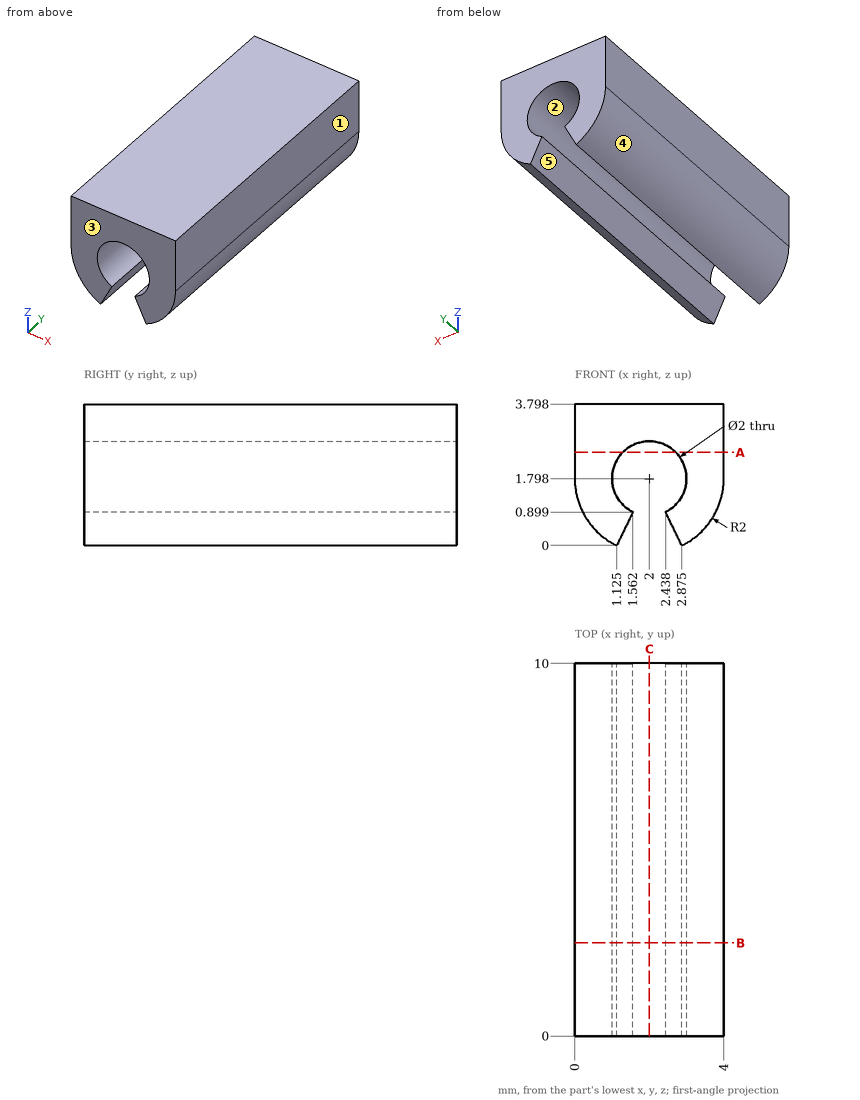
Print and shaded views of the part. All mm, measured from the part's lowest x, y and z. A direction names the side the tool comes from. Coordinates: 2 decimals unless noted, no trailing zeros. Loops run counter-clockwise (first coordinate to the right, second up) from the corner with the lowest first, then second, coordinate; pieces in that order, holes last. Notation, with made-up numbers: (22.25, 84.5) -> (57.25, 84.5) arc R27 ccw to (57.25, 107.5) -> close; hole circle Ø1 at (72, -8.75). An arc over 180 degrees is marked (long way). Use a Markdown table: item, result. Add a question column.
Item 1: Band-saw the part on B-B on y = 2.5. Write the cut outline in (x, z) (1 decimal).
Item 2: Band-saw the part on C-C on x = 2. Write the cut outline in (y, z).
Item 3: Probe probe 1 along X at (y, z) = (8.5, 1.45); probe 2 along X at (y, z) = (1.5, 2.7) (1 decimal); probe 3 along Z at (x, y) = (0.4, 3.5) (1 decimal). List the from-to ranges inside material, lowest first.
Item 4: Pull direction X, two halves, no side cores. Call the marked faces 1, 2 and 3: +X half, -X half, draft (parallel to the pull), parting line (faces both ways), or undercut.
Item 5: Band-saw the part on A-A on z = 2.5. Write the cut outline in (x, y).
Item 6: Which spindle directions (+Z, -Z, +X, -X, +Y, -Y) get a long thin tool onto all of the face, cutting with end or side? Do the marked faces 4 and 5. Say none if no direction does.
Geometry says:
| question | item | result |
|---|---|---|
| 1 | outline | (0, 1.8) arc R2 ccw to (1.1, 0) -> (1.6, 0.9) arc R1 cw (long way) to (2.4, 0.9) -> (2.9, 0) arc R2 ccw to (4, 1.8) -> (4, 3.8) -> (0, 3.8) -> close |
| 2 | outline | (0, 2.8) -> (10, 2.8) -> (10, 3.8) -> (0, 3.8) -> close |
| 3 | probe 1 | 0.03 to 1.06, 2.94 to 3.97 |
| 3 | probe 2 | 0 to 1.6, 2.4 to 4 |
| 3 | probe 3 | 0.6 to 3.8 |
| 4 | face 1 | +X half |
| 4 | face 2 | undercut |
| 4 | face 3 | draft |
| 5 | outline | (0, 0) -> (1.29, 0) -> (1.29, 10) -> (0, 10) -> close; (2.71, 0) -> (4, 0) -> (4, 10) -> (2.71, 10) -> close |
| 6 | face 4 | -Z, -X, +Y, -Y |
| 6 | face 5 | -Z, +Y, -Y |
